For this review, take the finished solid that the model builds, in its own axes (mm). A direction names the side the tool comes from. Coordinates: 2 decimals unless noted, no trailing zeros. Loops run counter-clockwise (first coordinate to the right, second up) from the corner with the lowest first, then second, coordinate; pieces in that order, holes last. Notation, with made-up numbers: (77, 59.25) -> (122, 59.25) arc R16 ccw to (122, 77.25) -> close; hole circle Ø3 at (49, 16.25). An arc over 180 degrees is marked (long way). Answer in a Markdown table with one row per item.
from build123d import *

# Parameters (mm, degrees)
SKETCH1_W           = 80
SKETCH1_H           = 75
BOSS_EXTRUDE1_DEPTH = 200
SHELL1_T            = -4


with BuildPart() as part:
    # Sketch1 → Boss-Extrude1 (new body)
    with BuildSketch(Plane.XY):
        with Locations((40, 37.5)):
            Rectangle(SKETCH1_W, SKETCH1_H)
    extrude(amount=-BOSS_EXTRUDE1_DEPTH)

    # Shell1
    shell1_openings = [part.faces().sort_by_distance(p)[0] for p in [
        (40, 75, -100),
    ]]
    offset(amount=SHELL1_T, openings=shell1_openings, kind=Kind.INTERSECTION)


solid = part.part
Item 1: Take a section at A-A, the plane y = 48. State the section outline as (x, z) points, and give its area (3 significant figures).
Worked answers:
| item | result |
|---|---|
| outline | (0, -200) -> (80, -200) -> (80, 0) -> (0, 0) -> close; hole (4, -196) -> (76, -196) -> (76, -4) -> (4, -4) -> close |
| area | 2,180 mm² |
Item 2: The part is to be moulded in two halves that separate along Z. For faces 3 (the flat face through (0, 37, -99)), 4 (the flat face through (39, 38, 0)), 5 (the flat face through (76, 39, -99)), say which applies: +Z half, -Z half, draft (parallel to the pull), parting line (faces both ways), or undercut.
Worked answers:
| item | result |
|---|---|
| face 3 | draft |
| face 4 | +Z half |
| face 5 | undercut |
Item 3: Take a section at B-B, the plane x = 33. State the section outline as (y, z) points.
Worked answers:
| item | result |
|---|---|
| outline | (0, -200) -> (75, -200) -> (75, -196) -> (4, -196) -> (4, -4) -> (75, -4) -> (75, 0) -> (0, 0) -> close |
Item 4: For L1, parallel to X at y = 59, z = -99; L2, parallel to Z at x = 33, y = 58; L3, parallel to Y at x = 54.5, z = -161.5, list the stretches that pass through material, from the lowest coordinate up.
Worked answers:
| item | result |
|---|---|
| L1 | 0 to 4, 76 to 80 |
| L2 | -200 to -196, -4 to 0 |
| L3 | 0 to 4 |
Item 5: Insertion check: pin 1 (1.5 mm diameter, centred on x = 22.5, z = -128.5, fed in from +Y). The pin has a flat end and moves straight along its axis. Give the tip position at first contact, or say it passes through.
Worked answers:
| item | result |
|---|---|
| pin 1 | y = 4 |
Item 6: Take a section at C-C, the plane z = -122. State the section outline as (x, y) points, and give its area (3 significant figures).
Worked answers:
| item | result |
|---|---|
| outline | (0, 0) -> (80, 0) -> (80, 75) -> (76, 75) -> (76, 4) -> (4, 4) -> (4, 75) -> (0, 75) -> close |
| area | 888 mm² |
Item 7: For faces 1 (the flat face through (80, 37, -99)), 2 (the flat face through (4, 39, -99)), list the 3-axis set-ups (+Z, -Z, +X, -X, +Y, -Y) from which the entire face can be reached by the end or side of a thin tool; tool diameter is ignored.
Worked answers:
| item | result |
|---|---|
| face 1 | +Z, -Z, +X, +Y, -Y |
| face 2 | +Y |
